The figure shows three views and two pictorial views of one solid part (mm, origin at its lowest corner). Answer the questions. A direction names the side the tool comes from. Give positions to 0.01 mm unless a question says otherwise; leave off trailing zeros. Write each loop counter-clockwise with the first axis right and the second up, starting at its lowest first coordinate (ties: lowest second). Pieces come first, ordered by that corner, then holes. Notation, with made-up numbers: (43, 58) -> (82, 58) arc R30 ccw to (82, 90) -> close; hole circle Ø2 at (-21, 45). An arc over 180 degrees is marked (long way). Use a Markdown table: item, result.
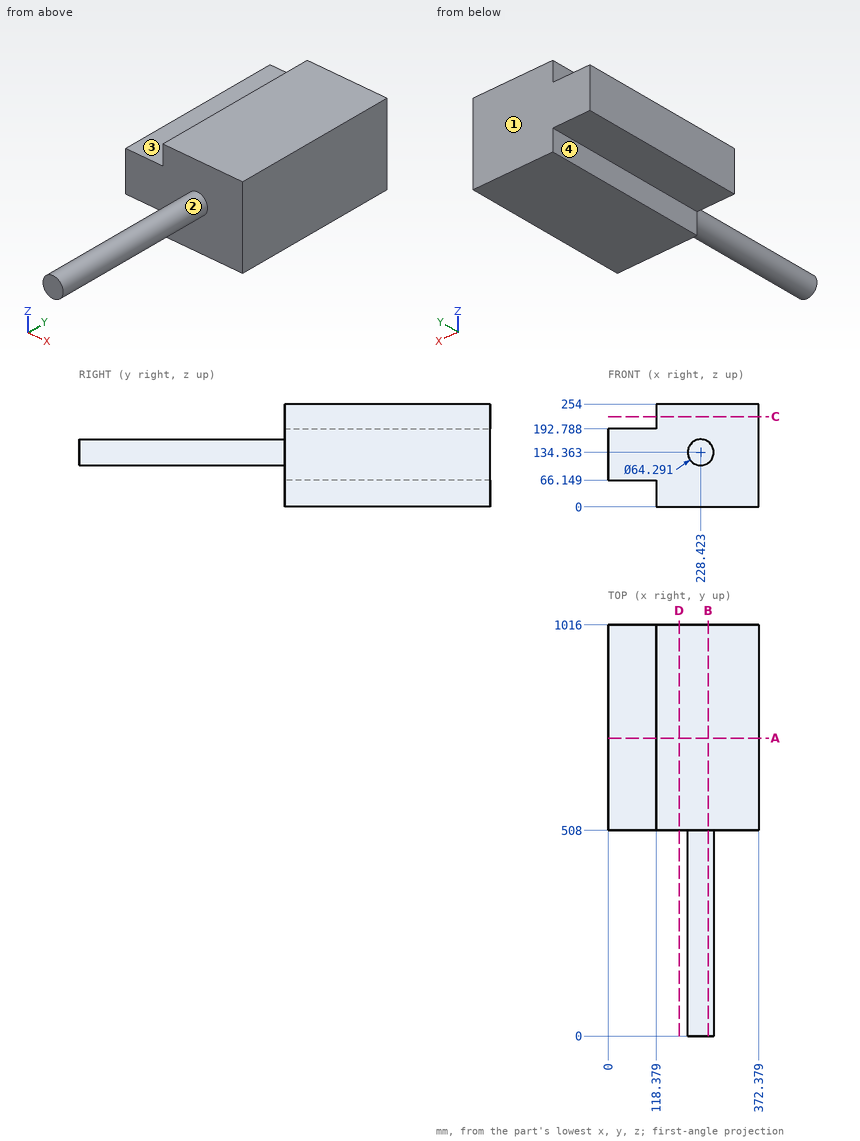
Item 1: A cutting plane is placed at B-B (x = 247). Give the vertices of the cut face in (y, z).
Return value:
| item | result |
|---|---|
| outline | (0, 108.13) -> (508, 108.13) -> (508, 0) -> (1016, 0) -> (1016, 254) -> (508, 254) -> (508, 160.6) -> (0, 160.6) -> close |
Item 2: A cutting plane is placed at A-A (y = 736). Give the vertices of the cut face in (x, z), then the cut area to 3 significant figures.
Return value:
| item | result |
|---|---|
| outline | (0, 66.15) -> (118.38, 66.15) -> (118.38, 0) -> (372.38, 0) -> (372.38, 254) -> (118.38, 254) -> (118.38, 192.79) -> (0, 192.79) -> close |
| area | 79,500 mm^2 |
Item 3: A cutting plane is placed at D-D (x = 175). Give the vertices of the cut face in (y, z), then the cut area to 3 significant figures.
Return value:
| item | result |
|---|---|
| outline | (508, 0) -> (1016, 0) -> (1016, 254) -> (508, 254) -> close |
| area | 129,000 mm^2 |
Item 4: Straight lines are drawn through the part: line 1 along Y through (x, z) = (130.5, 123.5); line 2 along X through (y, z) = (247.5, 136.5); line 3 along X through (y, z) = (955.5, 35.5). For each, find the intervals that lie inside material, in ascending order. Write a range as [from, to].
Return value:
| item | result |
|---|---|
| line 1 | [508, 1016] |
| line 2 | [196.35, 260.5] |
| line 3 | [118.38, 372.38] |
Item 5: A cutting plane is placed at C-C (z = 222.5). Give the vertices of the cut face in (x, y), then the cut area to 3 significant figures.
Return value:
| item | result |
|---|---|
| outline | (118.38, 508) -> (372.38, 508) -> (372.38, 1016) -> (118.38, 1016) -> close |
| area | 129,000 mm^2 |
Item 6: A tool of negligible diameter and unlimited length cuts with its end or side. For the marked faces 1, 2, 3 and 4, from which of +Z, -Z, +X, -X, +Y, -Y can it reach the whole face along a straight path? Write none if from no direction.
Return value:
| item | result |
|---|---|
| face 1 | +Z, -Z, +X, -X, +Y |
| face 2 | -Y |
| face 3 | +Z, -X, +Y, -Y |
| face 4 | -Z, -X, +Y, -Y |
Item 7: Each of these flat-tipped pins is pushed along its axis until it touches: P1, Ø1.5, axis at x = 190, z = 30, coming from the -Y side; P2, Ø1, axis at y = 445, z = 130, coming from the +X side (1 decimal). Where does it stop, or does it pass through?
Return value:
| item | result |
|---|---|
| P1 | y = 508 |
| P2 | x = 260.3 |
